The model under review builds one solid part; all positions refer to its coordinate system, in mm. A direction names the side the tool comes from. Coordinates: 2 decimals unless noted, no trailing zeros. Order: outer loops, then holes, each group sorted by start corner. A loop starts at its lowest first (then second) coordinate and runs counter-clockwise, first axis right, second up.
```python
from build123d import *

# Parameters (mm, degrees)
EXTRUDE_1_DEPTH     = 39
SKETCH_2_R          = 3.25
CUT_EXTRUDE_1_DEPTH = 9
SKETCH_3_R          = 3.25
CUT_EXTRUDE_2_DEPTH = 9


with BuildPart() as part:
    # Эскиз1 → Бобышка-Вытянуть1 (new body, symmetric)
    with BuildSketch(Plane.XY):
        Polygon((-78, 0), (0, 0), (0, 78), (-8, 78), (-8, 68.5), (-7.5, 68), (-8, 67.5), (-8, 54.5), (-7.5, 54), (-8, 53.5), (-8, 40.5), (-7.5, 40), (-8, 39.5), (-8, 30), (-30, 8), (-39.5, 8), (-40, 7.5), (-40.5, 8), (-53.5, 8), (-54, 7.5), (-54.5, 8), (-67.5, 8), (-68, 7.5), (-68.5, 8), (-78, 8), align=None)
        with BuildLine():
            Line((-4.5, 12), (-4.5, 26.136038969))
            ThreePointArc((-4.5, 26.136038969), (-5.117316568, 27.059918502), (-6.207106781, 26.843145751))
            Line((-6.207106781, 26.843145751), (-26.843145751, 6.207106781))
            ThreePointArc((-26.843145751, 6.207106781), (-27.059918502, 5.117316568), (-26.136038969, 4.5))
            Line((-26.136038969, 4.5), (-12, 4.5))
            Line((-12, 4.5), (-12, 7.9))
            ThreePointArc((-12, 7.9), (-14.899137803, 9.100862197), (-16.1, 12))
            ThreePointArc((-16.1, 12), (-15.1, 13), (-14.1, 12))
            ThreePointArc((-14.1, 12), (-10.51507576, 10.51507576), (-12, 14.1))
            ThreePointArc((-12, 14.1), (-13, 15.1), (-12, 16.1))
            ThreePointArc((-12, 16.1), (-9.100862197, 14.899137803), (-7.9, 12))
            Line((-7.9, 12), (-4.5, 12))
        make_face(mode=Mode.SUBTRACT)
    extrude(amount=EXTRUDE_1_DEPTH, both=True)

    # Эскиз2 → Вырез-Вытянуть1 (cut, through all)
    with BuildSketch(Plane.ZY.offset(8)):
        with Locations(Location((-20, 54, 0), (0, 0, 270))):  # turned: the seam where the file's is
            Circle(SKETCH_2_R)
        with Locations(Location((20, 54, 0), (0, 0, 270))):  # turned: the seam where the file's is
            Circle(SKETCH_2_R)
    extrude(amount=-CUT_EXTRUDE_1_DEPTH, mode=Mode.SUBTRACT)

    # Эскиз3 → Вырез-Вытянуть2 (cut, through all)
    with BuildSketch(Plane(origin=(0, 8, 0), x_dir=(1, 0, 0), z_dir=(0, 1, 0))):
        with Locations(Location((-54, -20, 0), (0, 0, 180))):  # turned: the seam where the file's is
            Circle(SKETCH_3_R)
        with Locations(Location((-54, 20, 0), (0, 0, 180))):  # turned: the seam where the file's is
            Circle(SKETCH_3_R)
    extrude(amount=-CUT_EXTRUDE_2_DEPTH, mode=Mode.SUBTRACT)


solid = part.part
```
(1) We need section D-D, the plane y = 43.5. Write out the cut boundary in (x, z), and give its area (3 significant figures).
A:
outline: (-8, -39) - (0, -39) - (0, 39) - (-8, 39) - close
area: 624 mm2
(2) We need section A-A, the plane z = -20. Count the separate pieces of the cut face and the enclosed holes in it, and give its area (3 significant figures).
A:
separate pieces: 3
enclosed holes: 1
area: 1,110 mm2
(3) For pin 1 Ø14.5 at (x, z) = (-61.5, -9) entering from +Y; pin 2 Ø3 at (y, z) = (58, 14) entering from -X; pin 3 Ø11.5 at (y, z) = (19.5, -13) entering from -X, all flat-tipped, find the tip position at first contact; note any pin that passes through.
A:
pin 1: stops at y = 8
pin 2: stops at x = -8
pin 3: stops at x = -24.25
(4) We need section B-B, the plane y = 52. Write out the cut boundary in (x, z).
A:
outline: (-8, -39) - (0, -39) - (0, -22.56) - (-8, -22.56) - close; (-8, -17.44) - (0, -17.44) - (0, 17.44) - (-8, 17.44) - close; (-8, 22.56) - (0, 22.56) - (0, 39) - (-8, 39) - close
(5) Machinability: for faces 1 (the face through (-8, 47, 1)), 2 (the face through (-19, 4.5, 1)), 3 (the face through (-53.295, 4.056, 16.827)), which of the approach directions +Z, -Z, +X, -X, +Y, -Y give a long, thin tool a straight path to every point of the face, cutting with its end or side? Answer none if there is none.
A:
face 1: +Z, -Z, -X, +Y
face 2: +Z, -Z
face 3: +Y, -Y
(6) We need section C-C, the plane y = 21. Write out the cut boundary in (x, z).
A:
outline: (-17, -39) - (-12.05, -39) - (-12.05, 39) - (-17, 39) - close; (-4.5, -39) - (0, -39) - (0, 39) - (-4.5, 39) - close
(7) Draft analysis for pull direction Y (two halves, no side actions). For faces 4 (the face through (-16.38, 16.67, 0.55)), 5 (the face through (-73, 8, 1)), 6 (the face through (0, 38, 1)), state which applies: released by +Y, released by -Y, zero draft, split by the parting line, or undercut.
A:
face 4: undercut
face 5: released by +Y
face 6: zero draft
(8) Wall thickness on probe 1 along Z at (x, y) = (-54, 6); probe 2 along X at (y, z) = (2, 20); probe 3 along X at (y, z) = (11.5, 31): over which ranges is each line inside the solid? List them lowest first.
A:
probe 1: z = -39 to -23.25, -16.75 to 16.75, 23.25 to 39
probe 2: x = -78 to -57.25, -50.75 to 0
probe 3: x = -26.5 to -21.55, -16.07 to -14.04, -9.96 to 0
